For this review, take the finished solid that the model builds, in its own axes (mm). Face numbers are marked on the shaded views. Round coordinates to 2 decimals unless told otherwise and drop trailing zeros. Loops run counter-clockwise (first coordinate to the right, second up) from the corner with the lowest first, then second, coordinate; pieces in that order, holes last. Notation, with made-up numbers: M 4.25,88.5 L 10.25,88.5 A21 cw 10.25,100.5 Z; hole C 68.5,54.5 d4. An arc over 180 degrees is marked long. Write item = value, one per line. Start each with the question number.
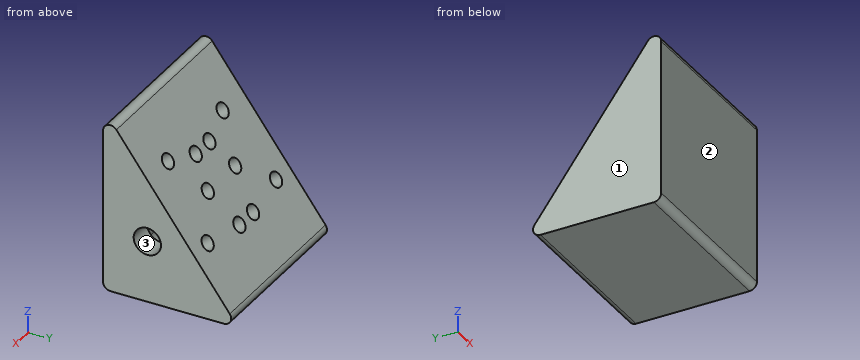
```python
from build123d import *

# Parameters (mm, degrees)
BOSS_EXTRUDE2_DEPTH      = 35
BOSS_EXTRUDE2_DEPTH_BACK = 35
FILLET1_R                = 3
CUT_EXTRUDE1_START       = -5
CUT_EXTRUDE1_DEPTH       = 60
SKETCH6_R                = 3.0734
CUT_EXTRUDE2_DEPTH       = 8
CUT_EXTRUDE3_REACH       = 72
SKETCH7_R                = 5.55625
SKETCH8_R                = 5.55625
BOSS_EXTRUDE3_DEPTH      = 10
FILLET2_R                = 1


with BuildPart() as part:
    # Sketch3 → Boss-Extrude2 (new body, two sides)
    with BuildSketch(Plane(origin=(0, 0, 0), x_dir=(0, 0, -1), z_dir=(1, 0, 0))) as boss_extrude2_sk:
        Polygon((0, 0), (0, 55), (-75, 0), align=None)
    extrude(amount=BOSS_EXTRUDE2_DEPTH)
    extrude(boss_extrude2_sk.sketch, amount=-BOSS_EXTRUDE2_DEPTH_BACK)

    # Fillet1
    fillet1_edges = [part.edges().sort_by_distance(p)[0] for p in [
        (0, 0, 75),
        (0, 55, 0),
        (0, 0, 0),
    ]]
    fillet(fillet1_edges, radius=FILLET1_R)

    # Sketch5 → Cut-Extrude1 (cut)
    with BuildSketch(Plane(origin=(35, 0, 0), x_dir=(0, 0, -1), z_dir=(1, 0, 0)).offset(CUT_EXTRUDE1_START)):
        with BuildLine():
            Line((-4, 40.172688191), (-4, 9))
            ThreePointArc((-4, 9), (-5.464466094, 5.464466094), (-9, 4))
            Line((-9, 4), (-52.962756624, 4))
            ThreePointArc((-52.962756624, 4), (-53.913126287, 4.688877031), (-53.554120287, 5.806404996))
            Line((-53.554120287, 5.806404996), (-5.591363664, 40.979093187))
            ThreePointArc((-5.591363664, 40.979093187), (-4.547984327, 41.064698186), (-4, 40.172688191))
        make_face()
    extrude(amount=-CUT_EXTRUDE1_DEPTH, mode=Mode.SUBTRACT)

    # Sketch6 → Cut-Extrude2 (cut)
    with BuildSketch(Plane(origin=(0, 35.765895954, 26.228323699), x_dir=(1, 0, 0), z_dir=(0, 0.806404996, 0.591363664))):
        with Locations(Location((5, 5, 0), (0, 0, 270))):  # turned: the seam where the file's is
            Circle(SKETCH6_R)
        with Locations(Location((5, -25, 0), (0, 0, 270))):  # turned: the seam where the file's is
            Circle(SKETCH6_R)
        with Locations(Location((20, -30, 0), (0, 0, 270))):  # turned: the seam where the file's is
            Circle(SKETCH6_R)
        with Locations(Location((10, -12, 0), (0, 0, 270))):  # turned: the seam where the file's is
            Circle(SKETCH6_R)
        with Locations(Location((25, 2, 0), (0, 0, 270))):  # turned: the seam where the file's is
            Circle(SKETCH6_R)
    cut_extrude2 = extrude(amount=-CUT_EXTRUDE2_DEPTH, mode=Mode.SUBTRACT)

    # Mirror1: Cut-Extrude2 across plane
    add(cut_extrude2.mirror(Plane(origin=(0, 0, 0), x_dir=(0, 0, 1), z_dir=(1, 0, 0))), mode=Mode.SUBTRACT)

    # Sketch7 → Cut-Extrude3 (cut, up to next)
    with BuildSketch(Plane(origin=(35, 0, 0), x_dir=(0, 0, -1), z_dir=(1, 0, 0)), mode=Mode.PRIVATE) as cut_extrude3_sk1:
        with Locations((-25, 18)):
            Circle(SKETCH7_R)
    cut_extrude3_tool1 = extrude(cut_extrude3_sk1.sketch, amount=-CUT_EXTRUDE3_REACH, mode=Mode.PRIVATE) & part.part
    add(cut_extrude3_tool1.solids().sort_by_distance((35, 18, 25))[0], mode=Mode.SUBTRACT)

    # Sketch8 → Boss-Extrude3 (add)
    with BuildSketch(Plane(origin=(35, 0, 0), x_dir=(0, 0, -1), z_dir=(1, 0, 0))):
        with BuildLine():
            Line((-22.719584828, 28.418397666), (-35.622064762, 18.956579048))
            Line((-35.622064762, 18.956579048), (-31.451239967, 13.269090691))
            ThreePointArc((-31.451239967, 13.269090691), (-20.269090691, 11.548760033), (-18.548760033, 22.730909309))
            Line((-18.548760033, 22.730909309), (-22.719584828, 28.418397666))
        make_face()
        with Locations((-25, 18)):
            Circle(SKETCH8_R, mode=Mode.SUBTRACT)
    extrude(amount=-BOSS_EXTRUDE3_DEPTH)

    # Fillet2
    fillet2_edges = [part.edges().sort_by_distance(p)[0] for p in [
        (30, 12.381492022, 44.588092525),
        (30, 25.574653487, 20.634172431),
        (25, 25.574653487, 20.634172431),
        (30, 11.548760033, 20.269090691),
        (25, 11.548760033, 20.269090691),
        (30, 16.112834869, 33.536652364),
        (25, 16.112834869, 33.536652364),
        (30, 4.688877031, 53.913126287),
        (30, 34.698745426, 14.155474246),
        (30, 41.064698186, 4.547984327),
        (30, 24.586344095, 4),
        (30, 5.464466094, 5.464466094),
        (30, 4, 30.981378312),
        (-30, 4.688877031, 53.913126287),
        (-30, 4, 30.981378312),
        (-30, 5.464466094, 5.464466094),
        (-30, 24.586344095, 4),
        (-30, 41.064698186, 4.547984327),
        (-30, 23.392749091, 29.572741975),
    ]]
    fillet(fillet2_edges, radius=FILLET2_R)


solid = part.part
```
(1) Draft analysis for pull direction Y (two halves, no side actions). For the marked faces 1, 2 and 3, state which applies: +Y half, -Y half, draft (parallel to the pull), parting line (faces both ways), or undercut.
(2) Wall thickness on L1, parallel to X at y = 26.5, z = 18; L2, parallel to Y at x = 28.25, z = 25; L3, parallel to Y at x = 28.5, z = 26.5: over which ranges is each line inside the solid? List them lowest first.
(3) Add section A-A on x = 11. Write out the cut boundary in (y, z), and give its area (3 significant figures).
(4) For pin 1 Ø1 at (x, z) = (-19, 59.5) entering from +Y; pin 2 Ø1 at (x, z) = (10.5, 44.5) entering from +Y; pin 3 Ø3 at (x, z) = (12.5, 46) entering from +Y, all flat-tipped, find the tip position at first contact; note any pin that passes through.
(5) Add section B-B on y = 34. Count the separate pieces of the cut face and the enclosed holes in it, and give its area (3 significant figures).
Answer sheet:
q1.face_1 = draft
q1.face_2 = -Y half
q1.face_3 = undercut
q2.L1 = -35 to -30, 30 to 35
q2.L2 = 0 to 4, 10 to 12.44, 23.56 to 36.67
q2.L3 = 0 to 4, 10.14 to 12.65, 23.35 to 35.57
q3.outline = M 0,3 A3 ccw 3,0 L 49.08,0 A3 ccw 51.5,4.77 L 30.39,33.56 L 23.94,28.83 L 40.98,5.59 A1 cw 40.17,4 L 9,4 A5 cw 4,9 L 4,52.96 A1 cw 5.81,53.55 L 20.5,33.52 L 26.95,38.25 L 5.42,67.61 A3 ccw 0,65.84 Z
q3.area = 1,010 mm²
q4.pin_1 = 11.73
q4.pin_2 = 22.73
q4.pin_3 = 22.37
q5.separate_pieces = 1
q5.enclosed_holes = 3
q5.area = 1,190 mm²
